Part model, mm, in its own coordinate system. A direction names the side the tool comes from. Coordinates: 2 decimals unless noted, no trailing zeros. One line per question, with ' | ' between items. Start each with the question number.
1) 3-axis set-ups, long thin cutter, end or side, ignore diameter. For faces 1 (the face through (0, -5, -6.502)), 2 (the face through (3.95, -5, 6)), 3 (the face through (-3.315, -5, 2)), 4 (the face through (3.315, -5, -2)), 5 (the face through (0, -9.398, -1)): which of +Z, -Z, +X, -X, +Y, -Y reach the whole face in a straight line?
2) Probe L1, parallel to Y at x = -1.5, z = -4; L2, parallel to X at y = -5.5, z = 0.25; L3, parallel to X at y = -3.25, z = 2.25. List the from-to ranges inside material, lowest first. Write a range as from..to.
3) Drop flat-ended pins along their axis: pin 1 (3 mm diameter, centred on x = -1, z = -2.5, fed in from -Y); pin 2 (0.5 mm diameter, centred on y = -6.5, z = -2.5, fed in from -X); pin 3 (1.5 mm diameter, centred on y = -1, z = -0.5, fed in from -X). Give the stop position or say it passes through.
4) Two-plate mould, pull along Z, no slides. Class faces 6 (the face through (3.95, -5, -6)), 7 (the face through (0, -5, 6.502)), 8 (the face through (3.696, -5, 4)): released by +Z, released by -Z, zero draft, split by the parting line, or undercut.
Autodesk Inventor part; units mm, degrees
ref_plane "rot_XY" through (0, 6.6675, 0) normal (1, 0, 0) x (0, 0, -1)
ref_plane "rot_YZ" through (0, 6.6675, 0) normal (0, 0, -1) x (0, 1, 0)
ref_plane "rot_ZX" through (0, 6.6675, 0) normal (0, 1, 0) x (1, 0, 0)
sketch "Sketch_2" plane through (0, -0.254, 0) normal (0, 1, 0) x (1, 0, 0)
  line L0 (-3.9497, -5.1435) -> (-3.9497, -6.3724)
  arc A0 (-3.9497, -6.3724) -> (-3.8197, -6.5024) centre (-3.8197, -6.3724) ccw
  line L1 (-3.8197, -6.5024) -> (3.8197, -6.5024)
  arc A1 (3.8197, -6.5024) -> (3.9497, -6.3724) centre (3.8197, -6.3724) ccw
  line L2 (3.9497, -6.3724) -> (3.9497, -5.1435)
  line L3 (3.9497, -5.1435) -> (3.6957, -5.1435)
  line L4 (3.6957, -5.1435) -> (3.6957, -2.9397)
  line L5 (3.6957, -2.9397) -> (3.3147, -2.8725)
  line L6 (3.3147, -2.8725) -> (3.3147, -1.8265)
  line L7 (3.3147, -1.8265) -> (3.6957, -1.7593)
  line L8 (3.6957, -1.7593) -> (3.6957, 1.7593)
  line L9 (3.6957, 1.7593) -> (3.3147, 1.8265)
  line L10 (3.3147, 1.8265) -> (3.3147, 2.8725)
  line L11 (3.3147, 2.8725) -> (3.6957, 2.9397)
  line L12 (3.6957, 2.9397) -> (3.6957, 5.1435)
  line L13 (3.6957, 5.1435) -> (3.9497, 5.1435)
  line L14 (3.9497, 5.1435) -> (3.9497, 6.3724)
  arc A2 (3.9497, 6.3724) -> (3.8197, 6.5024) centre (3.8197, 6.3724) ccw
  line L15 (3.8197, 6.5024) -> (-3.8197, 6.5024)
  arc A3 (-3.8197, 6.5024) -> (-3.9497, 6.3724) centre (-3.8197, 6.3724) ccw
  line L16 (-3.9497, 6.3724) -> (-3.9497, 5.1435)
  line L17 (-3.9497, 5.1435) -> (-3.6957, 5.1435)
  line L18 (-3.6957, 5.1435) -> (-3.6957, 2.9397)
  line L19 (-3.6957, 2.9397) -> (-3.3147, 2.8725)
  line L20 (-3.3147, 2.8725) -> (-3.3147, 1.8265)
  line L21 (-3.3147, 1.8265) -> (-3.6957, 1.7593)
  line L22 (-3.6957, 1.7593) -> (-3.6957, -1.7593)
  line L23 (-3.6957, -1.7593) -> (-3.3147, -1.8265)
  line L24 (-3.3147, -1.8265) -> (-3.3147, -2.8725)
  line L25 (-3.3147, -2.8725) -> (-3.6957, -2.9397)
  line L26 (-3.6957, -2.9397) -> (-3.6957, -5.1435)
  line L27 (-3.6957, -5.1435) -> (-3.9497, -5.1435)
extrude "Extrusion1" add sketch "Sketch_2" against normal blind 9.1694
sketch "Sketch_1" plane through (0, -9.4234, 0) normal (0, 1, 0) x (1, 0, 0)
  line L0 (-3.1877, 6.1184) -> (-3.1877, -6.1184)
  arc A0 (-3.1877, -6.1184) -> (-3.0577, -6.2484) centre (-3.0577, -6.1184) ccw
  line L1 (-3.0577, -6.2484) -> (3.0577, -6.2484)
  arc A1 (3.0577, -6.2484) -> (3.1877, -6.1184) centre (3.0577, -6.1184) ccw
  line L2 (3.1877, -6.1184) -> (3.1877, 6.1184)
  arc A2 (3.1877, 6.1184) -> (3.0577, 6.2484) centre (3.0577, 6.1184) ccw
  line L3 (3.0577, 6.2484) -> (-3.0577, 6.2484)
  arc A3 (-3.0577, 6.2484) -> (-3.1877, 6.1184) centre (-3.0577, 6.1184) ccw
extrude "Extrusion2" cut sketch "Sketch_1" along normal blind 0.0254
sketch "Sketch_7" plane through (0, -9.4234, 0) normal (0, 1, 0) x (1, 0, 0)
  line L0 (-0.9271, 5.0927) -> (-0.9271, 4.3053)
  line L1 (-0.9271, 4.3053) -> (0.9271, 4.3053)
  line L2 (0.9271, 4.3053) -> (0.9271, 5.0927)
  line L3 (0.9271, 5.0927) -> (-0.9271, 5.0927)
extrude "Extrusion3" cut sketch "Sketch_7" along normal blind 0.254
pattern_linear "Rectangular Pattern1" count 3 spacing 4.699 along (0, 0, 1) of "Extrusion3"
ref_plane "rot_XY" through (0, 6.6675, 0) normal (1, 0, 0) x (0, 0, -1)
ref_plane "rot_YZ" through (0, 6.6675, 0) normal (0, 0, -1) x (0, 1, 0)
ref_plane "rot_ZX" through (0, 6.6675, 0) normal (0, 1, 0) x (1, 0, 0)
ref_plane "to_cover_XY" through (0, -0.254, 0) normal (0, 1, 0) x (1, 0, 0)
ref_plane "to_cover_YZ" through (0, -0.254, 0) normal (1, 0, 0) x (0, 0, -1)
ref_plane "to_cover_ZX" through (0, -0.254, 0) normal (0, 0, -1) x (0, 1, 0)
ref_plane "to_terminals_XY" through (0, -9.4234, 0) normal (0, 1, 0) x (1, 0, 0)
ref_plane "to_terminals_YZ" through (0, -9.4234, 0) normal (1, 0, 0) x (0, 0, -1)
ref_plane "to_terminals_ZX" through (0, -9.4234, 0) normal (0, 0, -1) x (0, 1, 0)
properties part number "M20121SA2W13BR-switch"
Reported:
1) face 1: -Z, +X, -X, +Y, -Y | face 2: +Z, -Z, +X, +Y, -Y | face 3: -X, +Y, -Y | face 4: +X, +Y, -Y | face 5: -Y
2) L1: y = -9.4..-0.25 | L2: x = -3.7..3.7 | L3: x = -3.31..3.31
3) pin 1: stops at y = -9.4 | pin 2: stops at x = -3.31 | pin 3: stops at x = -3.7
4) face 6: zero draft | face 7: released by +Z | face 8: undercut
